The listing builds one solid part. Answer for the finished solid, in the listing's coordinates (mm). Round coordinates to 2 decimals unless told otherwise and drop trailing zeros. Order: outer loops, then holes, each group sorted by start corner. A loop starts at its lowest first (then second) coordinate and runs counter-clockwise, first axis right, second up. Notation, with made-up numbers: M 64.25,24 L 110.25,24 A31 ccw 110.25,54 Z; hole C 76,-12.5 d11. An arc over 180 degrees is marked long. Put each result on its own line as item: value. Start each with the question number.
1. The part is cut by section C-C (y = -15.75). Give the vertices of the cut face in (x, z), then the cut area to 3 significant figures.
2. The part is cut by section B-B (x = 313). Give the vertices of the cut face in (y, z) (3 decimals), then the cut area to 3 significant figures.
3. The part is cut by section A-A (z = 12). Give the vertices of the cut face in (x, y), then the cut area to 3 significant figures.
4. Consider line 1 (Y direction, x = 367, z = 18); line 2 (X direction, y = -17, z = 17); line 3 (Z direction, x = 473.5, y = -8.25) (3 decimals). Determine where each line is inside the solid, lowest interval first.
5. Each of these flat-tipped pins is pushed along its axis until it touches: pin 1 Ø1.9 at (x, y) = (295.5, -10) entering from +Z (3 decimals); pin 2 Ø1.9 at (x, z) = (-4.5, 9.5) entering from -Y; pin 3 Ø1 at (y, z) = (-6, 16) entering from -X. Where does it stop, or does it pass through?
from build123d import *

# Parameters (mm, degrees)
F0_W     = 19.05
F0_H     = 19.05
F1_DEPTH = 520.7
F3_DEPTH = 6.35
F5_DEPTH = 6.35
F7_DEPTH = 3.175


with BuildPart() as f1:
    # F0 (on Right) → F1 (new body)
    with BuildSketch(Plane.YZ):
        with Locations((-9.525, 9.525)):
            Rectangle(F0_W, F0_H)
    extrude(amount=F1_DEPTH)

    # F2 (on face) → F3 (join)
    with BuildSketch(Plane.YZ.offset(520.7)):
        with BuildLine():
            ThreePointArc((-7.9375, 15.875), (-9.525, 17.4625), (-11.1125, 15.875))
            Line((-11.1125, 15.875), (-11.1125, 3.175))
            ThreePointArc((-11.1125, 3.175), (-9.525, 1.5875), (-7.9375, 3.175))
            Line((-7.9375, 3.175), (-7.9375, 15.875))
        make_face()
    extrude(amount=F3_DEPTH)

    # F4 (on face) → F5 (join)
    with BuildSketch(Plane(origin=(0, 0, 0), x_dir=(0, -1, 0), z_dir=(-1, 0, 0))):
        with BuildLine():
            ThreePointArc((11.1125, 15.875), (9.525, 17.4625), (7.9375, 15.875))
            Line((7.9375, 15.875), (7.9375, 3.175))
            ThreePointArc((7.9375, 3.175), (9.525, 1.5875), (11.1125, 3.175))
            Line((11.1125, 3.175), (11.1125, 15.875))
        make_face()
    extrude(amount=F5_DEPTH)

    # F6 (on face) → F7 (cut)
    with BuildSketch(Plane.XY.offset(19.05)):
        with BuildLine():
            ThreePointArc((0, -6.35), (-3.175, -9.525), (0, -12.7))
            Line((0, -12.7), (520.7, -12.7))
            ThreePointArc((520.7, -12.7), (523.875, -9.525), (520.7, -6.35))
            Line((520.7, -6.35), (0, -6.35))
        make_face()
    extrude(amount=-F7_DEPTH, mode=Mode.SUBTRACT)


solid = f1.part
Resolved:
1. outline: M 0,0 L 520.7,0 L 520.7,19.05 L 0,19.05 Z
1. area: 9,920 mm2
2. outline: M -19.05,0 L 0,0 L 0,19.05 L -6.35,19.05 L -6.35,15.875 L -12.7,15.875 L -12.7,19.05 L -19.05,19.05 Z
2. area: 343 mm2
3. outline: M -6.35,-11.11 L 0,-11.11 L 0,-19.05 L 520.7,-19.05 L 520.7,-11.11 L 527.05,-11.11 L 527.05,-7.94 L 520.7,-7.94 L 520.7,0 L 0,0 L 0,-7.94 L -6.35,-7.94 Z
3. area: 9,960 mm2
4. line 1: -19.05 to -12.7, -6.35 to 0
4. line 2: 0 to 520.7
4. line 3: 0 to 15.875
5. pin 1: z = 15.875
5. pin 2: y = -11.11
5. pin 3: x = 0
